```python
from build123d import *

# Parameters (mm, degrees)
SCALE_1_SCALE = 0.1


with BuildPart() as part:
    # 草图1 one side → 旋转6 (revolve)
    with BuildSketch(Plane.XY, mode=Mode.PRIVATE) as revolve_6_sk:
        Polygon((-188.810566164, -8.557887153), (126.189433836, -8.557887153), (126.189433836, 754.802017268), (80.146848974, 754.802017268), (80.146848974, 737.812396498), (38.326244001, 737.812396498), (20.683176277, 703.0661449), (13.608822902, 703.0661449), (0, 689.457321998), (0, 494.076683139), (20.683176277, 465.32501722), (71.652038589, 465.32501722), (71.652038589, 452.909525118), (20.683176277, 452.909525118), (-103.471744737, 381.442112847), (-153.810566164, 381.442112847), (-153.810566164, 361.011582025), (-143.810566164, 361.011582025), (-143.810566164, 83.57948853), (-148.810566164, 83.57948853), (-148.810566164, 62.91133749), (-153.810566164, 62.91133749), (-153.810566164, 41.54424733), align=None)
    revolve(revolve_6_sk.sketch.rotate(Axis((126.189433836, 41.54424733, 0), (0, 1, 0)), 180), axis=Axis((126.189433836, 41.54424733, 0), (0, 1, 0)))

    # 草图2 → 切除-旋转1 (revolve, cut)
    with BuildSketch(Plane.XY):
        Polygon((-176.273470249, -8.557887153), (-140.148471815, 41.54424733), (-140.148471815, 56.139540799), (-131.681675308, 56.139540799), (-131.681675308, 76.742078968), (-121.803746049, 76.742078968), (-121.803746049, 364.305826939), (126.189433836, 364.305826939), (126.189433836, -8.557887153), align=None)
    revolve(axis=Axis((126.189433836, 364.305826939, 0), (0, -1, 0)), mode=Mode.SUBTRACT)


with BuildPart() as part_1:
    # 缩放比例1: scaled about (126.189433836, 394.552183872, 0)
    add(part.part.scale(SCALE_1_SCALE).moved(Location((113.570490452, 355.096965485, 0))))


solid = part_1.part
```
Input: part model. Units: mm. Frame: model coordinates. A direction names the side the tool comes from. Coordinates: 2 decimals unless noted, no trailing zeros. Write each loop counter-clockwise with the first axis right and the second up, starting at its lowest first coordinate (ties: lowest second). Pieces come first, ordered by that corner, then holes.
1) Section A-A on y = 375.5. Output: boundary loops of the cut face in (x, z), and give its area (3 significant figures).
2) Mould query, pull axis Z, two halves, no side actions, for faces 1 (the conical face through (114.87, 399.94, -0.5)), 2 (the cylindrical face through (145.196, 361.755, -17.428)), 3 (the flat face through (105.9, 363.455, 18.2)), 4 (the conical face through (147.464, 359.008, 16.313)). Classes: pulls with the +Z half, pulls with the -Z half, needs draft (parallel to the pull), parting line crosses it, or undercut.
3) Section B-B on y = 418. Output: boundary loops of the cut face in (x, z).
4) Material intervals for line 1 along Y through (x, z) = (132, -2); line 2 along Z through (x, y) = (142, 381); line 3 along Y through (x, z) = (124.5, -27), sorted ascending.
5) Pin query (flat end, axial travel): pin 1 Ø25 at (x, z) = (119, 2) entering from -Y; pin 2 Ø1.5 at (x, z) = (121, -4) entering from +Y; pin 3 Ø4 at (y, z) = (372, -21.5) entering from +X. Return the tip coordinate at first contact, or that it passes through.
6) Set-up query: faces 5 (the cylindrical face through (128.706, 401, 4.838)), 6 (the cylindrical face through (152.9, 360.3, -8.4)), 7 (the flat face through (140, 360.711, -22)). Return all of +Z, -Z, +X, -X, +Y, -Y with unobstructed straight access to the full face (end or side cutting, diameter ignored); none if empty.
Check result:
1. outline: circle Ø54 at (126.19, 0); hole circle Ø49.6 at (126.19, 0)
1. area: 358 mm2
2. face 1: parting line crosses it
2. face 2: undercut
2. face 3: needs draft
2. face 4: undercut
3. outline: circle Ø25.24 at (126.19, 0)
4. line 1: y = 391.53 to 400.39, 401.63 to 428.88
4. line 2: z = -21.89 to -19.11, 19.11 to 21.89
4. line 3: y = 358.67 to 363.45, 391.2 to 393.24
5. pin 1: stops at y = 391.53
5. pin 2: stops at y = 428.88
5. pin 3: stops at x = 144.86
6. face 5: none
6. face 6: +Y
6. face 7: -Y
